Can you work these out from the model? Positions are in its coordinate system, mm. A direction names the side the tool comes from. Coordinates: 2 decimals unless noted, no trailing zeros. Order: outer loops, then holes, each group sorted by start corner. A loop starts at its lowest first (then second) coordinate and runs counter-clockwise, first axis right, second up. Notation, with made-up numbers: M 79,78.25 L 106,78.25 A14 cw 106,97.25 Z; hole C 89,-29.75 d4. An arc over 180 degrees is marked long. Answer as a JSON object with one key per item and string values.
from build123d import *

# Parameters (mm, degrees)
F0_W     = 14.5
F0_H     = 6.6
F0_W_2   = 12.5
F0_H_2   = 4.6
F1_DEPTH = 12
F0_W_3   = 11.5
F0_H_3   = 1.7
F2_DEPTH = 2
F3_DEPTH = 10
F4_R     = 0.49999
F6_DEPTH = 0.4


# Not quite as in the source:
# - a fillet or chamfer is up to 0.001 mm smaller than in the source, because OpenCascade refuses the exact size


with BuildPart() as f1:
    # F0 (on Top) → F1 (new body)
    with BuildSketch(Plane.XY):
        with Locations((0.6113282288, 0)):
            Rectangle(F0_W, F0_H)
        with Locations((0.6113282288, 0)):
            Rectangle(F0_W_2, F0_H_2, mode=Mode.SUBTRACT)
    extrude(amount=F1_DEPTH)

    # F0 (on Top) → F2 (join)
    with BuildSketch(Plane.XY):
        with Locations((0.6113282288, 0)):
            Rectangle(F0_W_2, F0_H_2)
        with Locations((0.6113282288, 0.95)):
            Rectangle(F0_W_3, F0_H_3, mode=Mode.SUBTRACT)
        with Locations((0.6113282288, 0.95)):
            Rectangle(F0_W_3, F0_H_3)
    extrude(amount=F2_DEPTH)

    # F0 (on Top) → F3 (join)
    with BuildSketch(Plane.XY):
        with Locations((0.6113282288, 0.95)):
            Rectangle(F0_W_3, F0_H_3)
    extrude(amount=F3_DEPTH)

    # F4 (radius 0.5 in the source; OpenCascade refuses exactly that, so slightly less here)
    f4_edges = [f1.edges().sort_by_distance(p)[0] for p in [
        (-6.638672, 0, 12),
        (0.611328, -3.3, 12),
        (7.861328, 0, 12),
        (0.611328, 3.3, 12),
        (-5.638672, 0, 12),
        (0.611328, 2.3, 12),
        (6.861328, 0, 12),
        (0.611328, -2.3, 12),
        (7.861328, 3.3, 6),
        (7.861328, -3.3, 6),
        (7.861328, 0, 0),
        (0.611328, 3.3, 0),
        (-6.638672, 3.3, 6),
        (-6.638672, -3.3, 6),
        (0.611328, -3.3, 0),
        (-6.638672, 0, 0),
    ]]
    fillet(f4_edges, radius=F4_R)

    # F5 (on face) → F6 (cut)
    with BuildSketch(Plane(origin=(0, 3.3, 0), x_dir=(-1, 0, 0), z_dir=(0, 1, 0))):
        with BuildLine():
            Line((-4.1945352975, 7.1148852238), (-4.1945352975, 7.3648852238))
            ThreePointArc((-4.1945352975, 7.3648852238), (-6.193634283, 5.4249122664), (-4.3145352975, 3.3684884696))
            Line((-4.3145352975, 3.3684884696), (-4.3145352975, 3.6190043573))
            ThreePointArc((-4.3145352975, 3.6190043573), (-5.9435052109, 5.4249205618), (-4.1945352975, 7.1148852238))
        make_face()
        with BuildLine():
            Line((-4.3145352975, 3.6190043573), (-4.3145352975, 3.3684884696))
            ThreePointArc((-4.3145352975, 3.3684884696), (-4.1895255031, 3.3648914983), (-4.0645352975, 3.3691146959))
            Line((-4.0645352975, 3.3691146959), (-4.0645352975, 3.6197204751))
            ThreePointArc((-4.0645352975, 3.6197204751), (-4.1895224932, 3.6148924033), (-4.3145352975, 3.6190043573))
        make_face()
        with BuildLine():
            ThreePointArc((-4.0645352975, 3.3691146959), (-4.1895255031, 3.3648914983), (-4.3145352975, 3.3684884696))
            Line((-4.3145352975, 3.3684884696), (-4.3145352975, 1.8648852238))
            Line((-4.3145352975, 1.8648852238), (-4.0645352975, 1.8648852238))
            Line((-4.0645352975, 1.8648852238), (-4.0645352975, 3.3691146959))
        make_face()
        with BuildLine():
            Line((-4.0645352975, 3.6197204751), (-4.0645352975, 3.3691146959))
            ThreePointArc((-4.0645352975, 3.3691146959), (-2.7350833455, 3.9974057907), (-2.1945352975, 5.3648852238))
            Line((-2.1945352975, 5.3648852238), (-2.4445352975, 5.3648852238))
            ThreePointArc((-2.4445352975, 5.3648852238), (-2.4490283635, 5.2395634644), (-2.4624844899, 5.1148852238))
            ThreePointArc((-2.4624844899, 5.1148852238), (-3.000513644, 4.0855055729), (-4.0645352975, 3.6197204751))
        make_face()
        with BuildLine():
            Line((-4.3145352975, 5.3648852238), (-4.3145352975, 3.6190043573))
            ThreePointArc((-4.3145352975, 3.6190043573), (-4.1895224932, 3.6148924033), (-4.0645352975, 3.6197204751))
            Line((-4.0645352975, 3.6197204751), (-4.0645352975, 5.1148852238))
            Line((-4.0645352975, 5.1148852238), (-2.4624844899, 5.1148852238))
            ThreePointArc((-2.4624844899, 5.1148852238), (-2.4490283635, 5.2395634644), (-2.4445352975, 5.3648852238))
            Line((-2.4445352975, 5.3648852238), (-4.3145352975, 5.3648852238))
        make_face()
    extrude(amount=-F6_DEPTH, mode=Mode.SUBTRACT)


solid = f1.part
Item 1: I'm going to push flat-ended pins straight in: pin 1 (1.4 mm diameter, centred on x = -2.5, y = -0.5, fed in from +Z); pin 2 (1.5 mm diameter, centred on x = -4.5, y = 2.5, fed in from +Z). Where does each tip first touch, or does it pass through?
Answers follow:
{"pin 1": "stops at z = 10", "pin 2": "stops at z = 12"}
Item 2: Which directions (+Z, -Z, +X, -X, +Y, -Y) give clear straight access to the entire face, cutting with the end or side of a thin tool? Please do faces 4 (the cylindrical face through (2.75, 3.1, 3.98)), 5 (the flat face through (3.4, 3.3, 4.5)), 6 (the flat face through (1, -2.3, 7)).
Answers follow:
{"face 4": "+Y", "face 5": "+Z, -Z, +X, -X, +Y", "face 6": "+Z"}
Item 3: I want a section at A-A, the plane z = 8.5. Write out the boundary of the cut face in (x, y), plus the area to 3 significant figures.
Answers follow:
{"outline": "M -6.64,-2.8 A0.5 ccw -6.14,-3.3 L 7.36,-3.3 A0.5 ccw 7.86,-2.8 L 7.86,2.8 A0.5 ccw 7.36,3.3 L -6.14,3.3 A0.5 ccw -6.64,2.8 Z; M -5.14,0.1 L 6.36,0.1 L 6.36,1.8 L -5.14,1.8 Z; hole M -5.64,-2.3 L 6.86,-2.3 L 6.86,2.3 L -5.64,2.3 Z", "area": "57.5 mm^2"}
Item 4: If we mould it in two halves opening along Z, with no side actions, what happens to faces 1 (the flat face through (1, 1.8, 6)), 2 (the cylindrical face through (2.988, 3.103, 4.097)), 3 (the flat face through (1, 0, 0))? For each: pulls with the +Z half, pulls with the -Z half, needs draft (parallel to the pull), parting line crosses it, or undercut.
Answers follow:
{"face 1": "needs draft", "face 2": "undercut", "face 3": "pulls with the -Z half"}
Item 5: Please list where these lines run through material, in increasing order: line 1 (Y direction, x = 3, z = 2.75); line 2 (X direction, y = 1.25, z = 6); line 3 (X direction, y = -2.25, z = 5).
Answers follow:
{"line 1": "y = -3.3 to -2.3, 0.1 to 1.8, 2.3 to 3.3", "line 2": "x = -6.64 to -5.64, -5.14 to 6.36, 6.86 to 7.86", "line 3": "x = -6.64 to -5.64, 6.86 to 7.86"}
Item 6: I want a section at B-B, the plane z = 10.5. Write out the boundary of the cut face in (x, y), plus the area to 3 significant figures.
Answers follow:
{"outline": "M -6.64,-2.8 A0.5 ccw -6.14,-3.3 L 7.36,-3.3 A0.5 ccw 7.86,-2.8 L 7.86,2.8 A0.5 ccw 7.36,3.3 L -6.14,3.3 A0.5 ccw -6.64,2.8 Z; hole M -5.64,-2.3 L 6.86,-2.3 L 6.86,2.3 L -5.64,2.3 Z", "area": "38.0 mm^2"}
